The figure shows three views and two pictorial views of one solid part (mm, origin at its lowest corner). Answer the questions. A direction names the side the tool comes from. Coordinates: 2 decimals unless noted, no trailing zeros. Order: outer loops, then holes, each group sorted by start corner. A loop starts at its lowest first (then second) coordinate and runs counter-clockwise, first axis right, second up. Notation, with made-up numbers: (-1.75, 51) -> (44.25, 51) arc R12 cw to (44.25, 69) -> close; hole circle Ø8 at (-0.5, -22). An arc over 180 degrees is marked (long way). Return JSON: item names as keys, results as strings.
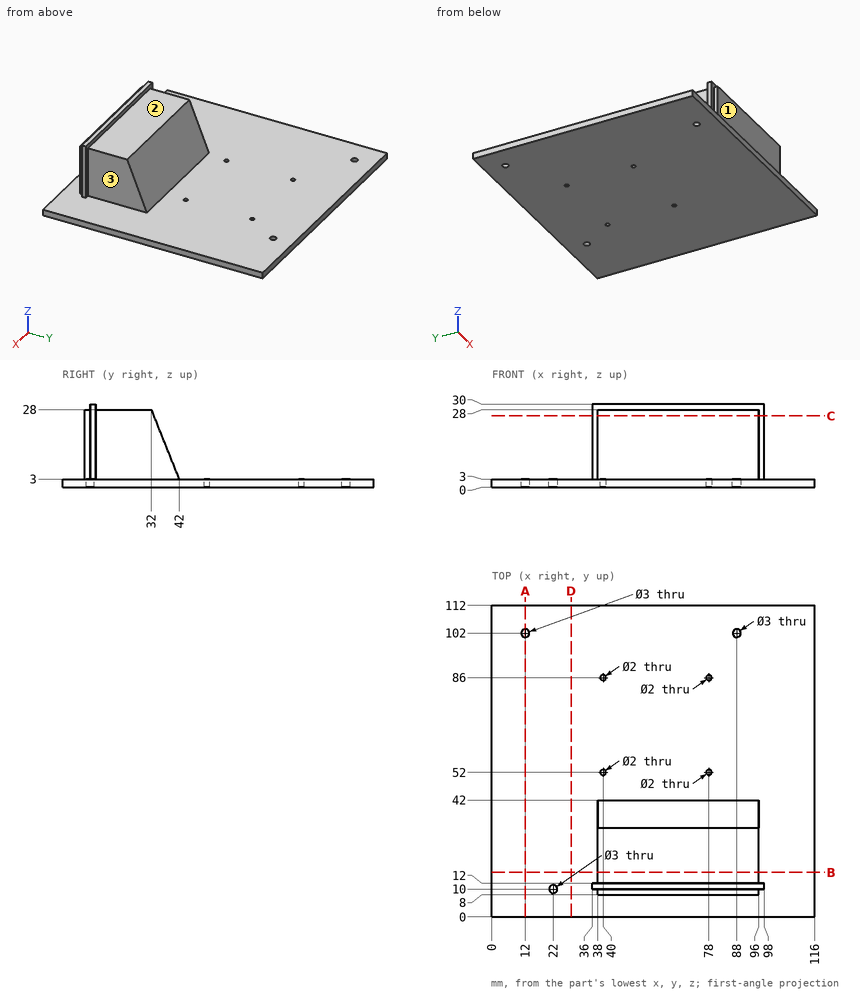
1. For the marked faces 1, 2 and 3, determine the directions among +Z, -Z, +X, -X, +Y, -Y from which every point of the face is accessible in a straight line to the end or side of a thin tool.
Answer block:
{"face 1": "+Z, +X, -X, -Y", "face 2": "+Z, +X, -X, +Y", "face 3": "+Z, +X, +Y"}
2. The part is cut by section C-C on z = 25.75. Give the vertices of the cut face in (x, y).
Answer block:
{"outline": "(36, 10) -> (38, 10) -> (38, 8) -> (96, 8) -> (96, 10) -> (98, 10) -> (98, 12) -> (96, 12) -> (96, 32.9) -> (38, 32.9) -> (38, 12) -> (36, 12) -> close"}
3. Consider line 1 (Y direction, x = 78, z = 1.4); line 2 (X direction, y = 86, z = 1.85); line 3 (X direction, y = 102, z = 1.8). Determine where each line is inside the solid, lowest interval first. Write a range as from..to.
Answer block:
{"line 1": "y = 0..51, 53..85, 87..112", "line 2": "x = 0..39, 41..77, 79..116", "line 3": "x = 0..10.5, 13.5..86.5, 89.5..116"}
4. Each of these flat-tipped pins is pushed along its axis until it touches: pin 1 Ø4 at (x, z) = (77.5, 24.5) entering from -Y; pin 2 Ø1.8 at (x, y) = (40, 52) entering from -Z; pin 3 Ø3.5 at (x, y) = (12, 102) entering from +Z; pin 4 Ø2 at (y, z) = (9.5, 10.5) entering from +X. Where does it stop, or does it pass through?
Answer block:
{"pin 1": "stops at y = 8", "pin 2": "passes through", "pin 3": "stops at z = 3", "pin 4": "stops at x = 98"}
5. The part is cut by section B-B on y = 16. Give the vertices of the cut face in (x, z), and give its area (3 significant figures).
Answer block:
{"outline": "(0, 0) -> (116, 0) -> (116, 3) -> (96, 3) -> (96, 28) -> (38, 28) -> (38, 3) -> (0, 3) -> close", "area": "1,800 mm2"}
6. The part is cut by section A-A on x = 12. Give the vertices of the cut face in (y, z).
Answer block:
{"outline": "(0, 0) -> (100.5, 0) -> (100.5, 3) -> (0, 3) -> close; (103.5, 0) -> (112, 0) -> (112, 3) -> (103.5, 3) -> close"}
7. The part is cut by section D-D on x = 28.5. Give the vertices of the cut face in (y, z), and give its area (3 significant figures).
Answer block:
{"outline": "(0, 0) -> (112, 0) -> (112, 3) -> (0, 3) -> close", "area": "336 mm2"}
